The model under review builds one solid part; all positions refer to its coordinate system, in mm. Face numbers are marked on the shaded views. A direction names the side the tool comes from. Coordinates: 2 decimals unless noted, no trailing zeros. Write each loop counter-clockwise with the first axis right and the second up, starting at its lowest first coordinate (ties: lowest second). Pieces come first, ordered by that corner, then holes.
1) Add section A-A, the plane x = 0. State the section outline as (y, z) points, then the cut area to 3 significant figures.
2) Machinability: for the marked faces 1 and 2, which of the approach directions +Z, -Z, +X, -X, +Y, -Y give a long, thin tool a straight path to every point of the face, cutting with its end or side? Answer none if there is none.
3) For P1, Ø12, axis at y = -4.5, z = 44.5, coming from the +X side; P2, Ø8, axis at x = -88.5, y = -73.5, coming from the +Z side; P3, Ø6, axis at x = 60.5, z = 20, coming from the -Y side; P4, Ø20, axis at x = 0, y = 0, coming from the -Z side, all flat-tipped, find the tip position at first contact; note any pin that passes through.
4) Mouldability with a two-part tool opening along Y and no side actions: class the marked faces 3, 4 and 5 as released by +Y, released by -Y, zero draft, split by the parting line, or undercut.
5) Add section D-D, the plane z = 5.5. State the section outline as (x, y) points.
6) Add section C-C, the plane z = 56. State the section outline as (x, y) points.
7) For line 1 (Y direction, x = 0, z = 46.5); line 2 (Z direction, x = 75.5, y = -61); line 3 (Y direction, x = -18, z = 42.5), list the stretches that pass through material, from the lowest coordinate up.
from build123d import *

# Parameters (mm, degrees)
F3_D           = 22
F3_CBORE_D     = 50
F3_CBORE_DEPTH = 30
F4_R           = 10


with BuildPart() as f1:
    # F0 (on Front) → F1 (revolve)
    with BuildSketch(Plane.XZ):
        Polygon((0, 60), (0, 0), (130, 0), (109.792741, 35), (60, 35), (60, 60), align=None)
    revolve(axis=Axis((0, 0, 30), (0, 0, 1)))

    # F3 (through all)
    with Locations(Plane.XY.offset(60)):
        with Locations((0, 0)):
            CounterBoreHole(F3_D / 2, F3_CBORE_D / 2, F3_CBORE_DEPTH)

    # F4
    f4_edges = [f1.edges().sort_by_distance(p)[0] for p in [
        (-60, 0, 35),
        (-109.792741, 0, 35),
    ]]
    fillet(f4_edges, radius=F4_R)


solid = f1.part
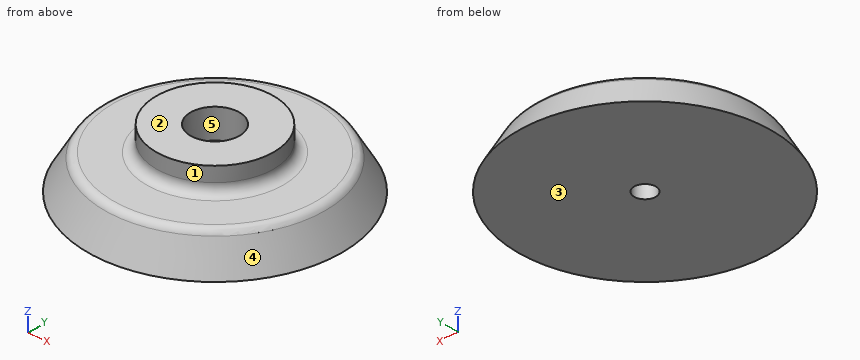
Geometry results:
1. outline: (-130, 0) - (-11, 0) - (-11, 30) - (-25, 30) - (-25, 60) - (-60, 60) - (-60, 45) arc R10 cw to (-70, 35) - (-104.02, 35) arc R10 ccw to (-112.68, 30) - close; (11, 0) - (130, 0) - (112.68, 30) arc R10 ccw to (104.02, 35) - (70, 35) arc R10 cw to (60, 45) - (60, 60) - (25, 60) - (25, 30) - (11, 30) - close
1. area: 9,260 mm2
2. face 1: +Z
2. face 2: +Z, +X, -X, +Y, -Y
3. P1: stops at x = 62.25
3. P2: stops at z = 32.12
3. P3: stops at y = -104.48
3. P4: passes through
4. face 3: zero draft
4. face 4: split by the parting line
4. face 5: undercut
5. outline: circle Ø253.65 at (0, 0); hole circle Ø22 at (0, 0)
6. outline: circle Ø120 at (0, 0); hole circle Ø50 at (0, 0)
7. line 1: y = -60 to -25, 25 to 60
7. line 2: z = 0 to 35
7. line 3: y = -57.57 to -17.35, 17.35 to 57.57
